```python
from build123d import *

# Parameters (mm, degrees)
F0_W     = 50
F0_H     = 50
F1_DEPTH = 25
F3_DEPTH = 25


with BuildPart() as f1:
    # F0 (on Front) → F1 (new body, symmetric)
    with BuildSketch(Plane.XZ):
        Rectangle(F0_W, F0_H)
    extrude(amount=F1_DEPTH, both=True)

    # F2 (on face) → F3 (cut)
    with BuildSketch(Plane(origin=(0, 25, 0), x_dir=(-1, 0, 0), z_dir=(0, 1, 0))):
        Polygon((15, 0), (0, 7.808506), (-15, 0), (0, -7.808506), align=None)
    extrude(amount=-F3_DEPTH, mode=Mode.SUBTRACT)


solid = f1.part
```
The model under review builds one solid part; all positions refer to its coordinate system, in mm. A direction names the side the tool comes from. Give positions to 0.01 mm unless a question says otherwise; leave off trailing zeros. Loops run counter-clockwise (first coordinate to the right, second up) from the corner with the lowest first, then second, coordinate; pieces in that order, holes last. Notation, with made-up numbers: (-12.5, 17) - (-8.5, 17) arc R24 ccw to (-8.5, 40) - close; hole circle Ø11 at (-9, -38). An arc over 180 degrees is marked (long way). Answer as a JSON object with one key per item and string values.
Q1. To check wall thickness, follow line 1 along X through (y, z) = (3.5, 3.5); line 2 along Z through (x, y) = (9, 1); line 3 along Z through (x, y) = (13, 2). State the ranges of each line that lie inside material, in increasing order.
Worked out:
{"line 1": "x = -25 to -8.28, 8.28 to 25", "line 2": "z = -25 to -3.12, 3.12 to 25", "line 3": "z = -25 to -1.04, 1.04 to 25"}
Q2. Insertion check: pin 1 (4.5 mm diameter, centred on x = -4, z = -3, fed in from +Y). The pin has a flat end and moves straight along its axis. Give the tip position at first contact, or say it passes through.
Worked out:
{"pin 1": "stops at y = 0"}
Q3. Add section B-B on x = -3.5. State the section outline as (y, z) points, plus the area to 3 significant figures.
Worked out:
{"outline": "(-25, -25) - (25, -25) - (25, -5.99) - (0, -5.99) - (0, 5.99) - (25, 5.99) - (25, 25) - (-25, 25) - close", "area": "2,200 mm^2"}
Q4. Mouldability with a two-part tool opening along X and no side actions: class faces 3 (the flat face through (0, 0, -25)), 4 (the flat face through (25, 0, 0)), 5 (the flat face through (7.395, 12.675, 3.959)), 6 (the flat face through (-25, 0, 0)) as +X half, -X half, draft (parallel to the pull), parting line (faces both ways), or undercut.
Worked out:
{"face 3": "draft", "face 4": "+X half", "face 5": "undercut", "face 6": "-X half"}
Q5. Add section A-A on z = 1. State the section outline as (x, y) points, plus the area to 3 significant figures.
Worked out:
{"outline": "(-25, -25) - (25, -25) - (25, 25) - (13.08, 25) - (13.08, 0) - (-13.08, 0) - (-13.08, 25) - (-25, 25) - close", "area": "1,850 mm^2"}
Q6. For faces 1 (the flat face through (-6, 25, 6)), 2 (the flat face through (7.6, 12.68, -3.85)), list the 3-axis set-ups (+Z, -Z, +X, -X, +Y, -Y) from which the entire face can be reached by the end or side of a thin tool; tool diameter is ignored.
Worked out:
{"face 1": "+Z, -Z, +X, -X, +Y", "face 2": "+Y"}
